```python
from build123d import *

# Parameters (mm, degrees)
BOX_W                                = 57.2
BOX_H                                = 21.34
BOX_DEPTH                            = 2.79
BOX001_W                             = 51.2
BOX001_H                             = 15.16
BOX001_DEPTH                         = 10
BOX002_W                             = 4
BOX002_H                             = 15.16
BOX002_DEPTH                         = 0.92
BOX003_W                             = 4
BOX003_H                             = 15.16
BOX003_DEPTH                         = 0.92
CYLINDER_W                           = 1.025
CYLINDER_H                           = 5
CYLINDER_ANGLE                       = 180
CYLINDER001_R                        = 0.4
CYLINDER001_DEPTH                    = 0.25
CYLINDER002_R                        = 0.3105
CYLINDER002_DEPTH                    = 10
LINEARPATTERN_COUNT                  = 32
LINEARPATTERN_PITCH                  = 1.778065
CYLINDER003_R                        = 0.3105
CYLINDER003_DEPTH                    = 10
LINEARPATTERN001_COUNT               = 32
LINEARPATTERN001_PITCH               = 1.778065
CYLINDER008_W                        = 1.55
CYLINDER008_H                        = 1.87
CYLINDER008_ANGLE                    = 180
CYLINDER008_LINEARPATTERN002_2_W     = 1.55
CYLINDER008_LINEARPATTERN002_2_H     = 1.87
CYLINDER008_LINEARPATTERN002_2_ANGLE = 180


with BuildPart() as part:
    # Box → Box (join)
    with BuildSketch(Plane(origin=(-28.6, -10.67, 2.8), x_dir=(1, 0, 0), z_dir=(0, 0, 1))):
        with Locations((28.6, 10.67)):
            Rectangle(BOX_W, BOX_H)
    extrude(amount=BOX_DEPTH)

    # Box001 → Box001 (cut)
    with BuildSketch(Plane(origin=(-25.6, -7.58, 0), x_dir=(1, 0, 0), z_dir=(0, 0, 1))):
        with Locations((25.6, 7.58)):
            Rectangle(BOX001_W, BOX001_H)
    extrude(amount=BOX001_DEPTH, mode=Mode.SUBTRACT)

    # Box002 → Box002 (cut)
    with BuildSketch(Plane(origin=(-29.16, -7.58, 4.67), x_dir=(1, 0, 0), z_dir=(0, 0, 1))):
        with Locations((2, 7.58)):
            Rectangle(BOX002_W, BOX002_H)
    extrude(amount=BOX002_DEPTH, mode=Mode.SUBTRACT)

    # Box003 → Box003 (cut)
    with BuildSketch(Plane(origin=(25, -7.58, 4.67), x_dir=(1, 0, 0), z_dir=(0, 0, 1))):
        with Locations((2, 7.58)):
            Rectangle(BOX003_W, BOX003_H)
    extrude(amount=BOX003_DEPTH, mode=Mode.SUBTRACT)

    # Cylinder → Cylinder (revolve, cut)
    with BuildSketch(Plane(origin=(-28.6, -4, 0), x_dir=(0, -1, 0), z_dir=(-1, 0, 0))):
        with Locations((0.5125, 2.5)):
            Rectangle(CYLINDER_W, CYLINDER_H)
    revolve(axis=Axis((-28.6, -4, 0), (0, 0, 1)), revolution_arc=CYLINDER_ANGLE, mode=Mode.SUBTRACT)

    # Cylinder001 → Cylinder001 (join)
    with BuildSketch(Plane(origin=(-27.559, -6.425, 4.67), x_dir=(1, 0, 0), z_dir=(0, 0, 1))):
        Circle(CYLINDER001_R)
    extrude(amount=CYLINDER001_DEPTH)

    # Cylinder002 → Cylinder002 (cut)
    with BuildSketch(Plane(origin=(-27.559, -9.525, 0), x_dir=(1, 0, 0), z_dir=(0, 0, 1))):
        Circle(CYLINDER002_R)
    cylinder002 = extrude(amount=CYLINDER002_DEPTH, mode=Mode.SUBTRACT)

    # LinearPattern: Cylinder002 ×32
    with Locations(*[(i * LINEARPATTERN_PITCH, 0, 0) for i in range(1, LINEARPATTERN_COUNT)]):
        add(cylinder002, mode=Mode.SUBTRACT)

    # Cylinder003 → Cylinder003 (cut)
    with BuildSketch(Plane(origin=(-27.559, 9.525, 0), x_dir=(1, 0, 0), z_dir=(0, 0, 1))):
        Circle(CYLINDER003_R)
    cylinder003 = extrude(amount=CYLINDER003_DEPTH, mode=Mode.SUBTRACT)

    # LinearPattern001: Cylinder003 ×32
    with Locations(*[(i * LINEARPATTERN001_PITCH, 0, 0) for i in range(1, LINEARPATTERN001_COUNT)]):
        add(cylinder003, mode=Mode.SUBTRACT)

    # Cylinder008 → Cylinder008 (revolve)
    with BuildSketch(Plane(origin=(-11.5, 7.6, 2.8), x_dir=(-1, 0, 0), z_dir=(0, 1, 0))):
        with Locations((0.775, 0.935)):
            Rectangle(CYLINDER008_W, CYLINDER008_H)
    cylinder008 = revolve(axis=Axis((-11.5, 7.6, 2.8), (0, 0, 1)), revolution_arc=CYLINDER008_ANGLE)

    # Cylinder008 LinearPattern002 2 → Cylinder008 LinearPattern002 2 (revolve)
    with BuildSketch(Plane(origin=(11.5, 7.6, 2.8), x_dir=(-1, 0, 0), z_dir=(0, 1, 0))):
        with Locations((0.775, 0.935)):
            Rectangle(CYLINDER008_LINEARPATTERN002_2_W, CYLINDER008_LINEARPATTERN002_2_H)
    cylinder008_linearpattern002_2 = revolve(axis=Axis((11.5, 7.6, 2.8), (0, 0, 1)), revolution_arc=CYLINDER008_LINEARPATTERN002_2_ANGLE)

    # Mirrored: Cylinder008, Cylinder008 LinearPattern002 2 across XZ
    add(cylinder008.mirror(Plane.XZ))
    add(cylinder008_linearpattern002_2.mirror(Plane.XZ))


solid = part.part
```
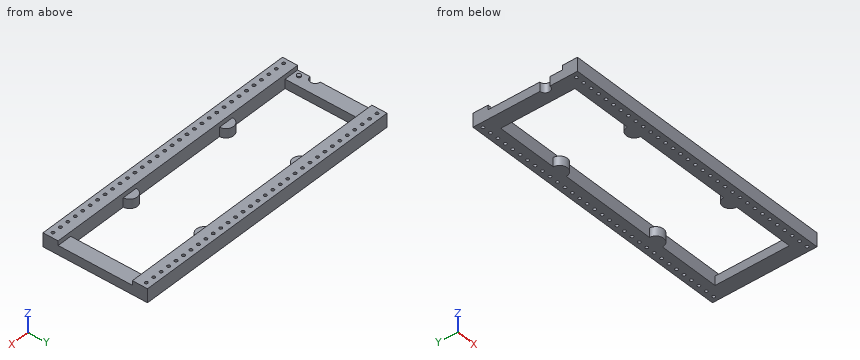
Read the model definition and answer for the solid it produces. Units are mm, in the model's axes. Give positions to 0.01 mm unless a question says otherwise; leave off trailing zeros. Write each loop counter-clockwise with the first axis right and the second up, starting at its lowest first coordinate (ties: lowest second). Pieces come first, ordered by that corner, then holes. Notation, with made-up numbers: M -1,5 L 49,5 A20 ccw 49,24 Z; hole C 13.25,8 d5. An arc over 180 degrees is marked long. Put each result on its own line as item: value. Start each with the question number.
1. The part is cut by section A-A, the plane y = -4. Give the vertices of the cut face in (x, z) (3 decimals), and give its area (3 significant figures).
2. The part is cut by section C-C, the plane z = 4.1. Give the number of separate pieces and of enclosed holes in the cut face, and give its area (3 significant figures).
3. Consider line 1 along Y through (x, z) = (24, 3.75); line 2 along X through (y, z) = (6.5, 4.05); line 3 along Y through (x, z) = (20, 3.5). Determine where each line is inside the solid, lowest interval first.
4. The part is cut by section B-B, the plane y = 0.5. Give the vertices of the cut face in (x, z), and give its area (3 significant figures).
5. Each of these flat-tipped pins is pushed along its axis until it touches: pin 1 Ø1 at (y, z) = (-6, 5) entering from +X; pin 2 Ø0.8 at (x, y) = (-11.5, -6.5) entering from +Z. Where does it stop, or does it pass through?
Final values:
1. outline: M -27.575,2.8 L -25.6,2.8 L -25.6,4.67 L -27.575,4.67 Z; M 25.6,2.8 L 28.6,2.8 L 28.6,4.67 L 25.6,4.67 Z
1. area: 9.30 mm²
2. separate pieces: 1
2. enclosed holes: 65
2. area: 438 mm²
3. line 1: y = -10.67 to -9.84, -9.21 to -7.58, 7.58 to 9.21, 9.84 to 10.67
3. line 2: x = -28.6 to -25.6, -12.59 to -10.41, 10.41 to 12.59, 25.6 to 28.6
3. line 3: y = -10.67 to -7.58, 7.58 to 10.67
4. outline: M -28.6,2.8 L -25.6,2.8 L -25.6,4.67 L -28.6,4.67 Z; M 25.6,2.8 L 28.6,2.8 L 28.6,4.67 L 25.6,4.67 Z
4. area: 11.2 mm²
5. pin 1: stops at x = 28.6
5. pin 2: stops at z = 4.67
